Check sheet for the modelled part. Datum: model origin and axes. Units: mm. Coordinates: 2 decimals unless noted, no trailing zeros. Order: outer loops, then holes, each group sorted by start corner. A loop starts at its lowest first (then second) coordinate and runs counter-clockwise, first axis right, second up.
1. Gauge pin test, flat ends, axial feed: pin 1 Ø3 at (x, z) = (46.65, -18) entering from +Y; pin 2 Ø1 at (y, z) = (0.5, 15.5) entering from -X. Record the tip position at first contact, or that the pin passes through.
2. Cross-section at A-A (z = -6). Enter the section's corners in (x, y), then the cut area to 3 significant figures.
3. Thickness scan on line 1 (Z direction, x = 0, y = 1.45); line 2 (X direction, y = 1.35, z = 11.5); line 3 (Z direction, x = 34, y = 0.65). Record the ranges inside material, lowest first.
4. Cross-section at D-D (z = 23). Enter the section's corners in (x, y).
5. Cross-section at C-C (x = 0). Enter the section's corners in (y, z), then the cut area to 3 significant figures.
6. Cross-section at B-B (y = 0.3). Enter the section's corners in (x, z).
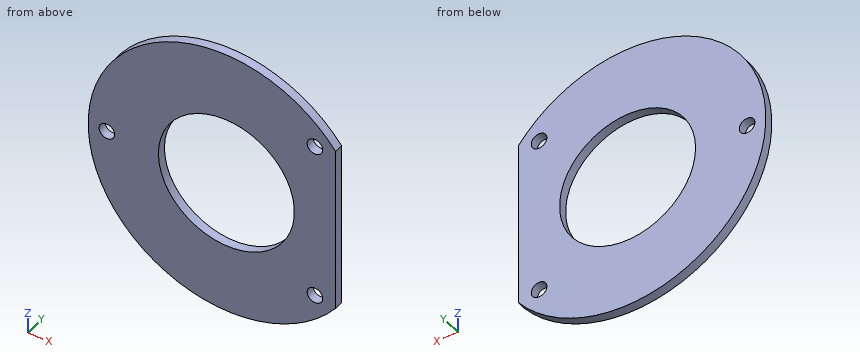
Autodesk Inventor part; units mm, degrees
ref_plane "YZ Plane" through (0, 0, 0) normal (1, 0, 0) x (0, 1, 0)
ref_plane "XZ Plane" through (0, 0, 0) normal (0, 1, 0) x (-1, 0, 0)
ref_plane "XY Plane" through (0, 0, 0) normal (0, 0, 1) x (1, 0, 0)
sketch "Sketch1" plane through (0, 0, 0) normal (0, 1, 0) x (-1, 0, 0)
  circle A0 centre (0, 0) radius 1.75
  line L0 (0, 0) -> (-46.6476, -18) construction
  line L1 (-46.6476, -18) -> (-46.6476, 18) construction
  line L2 (-46.6476, 18) -> (0, 0) construction
  circle A1 centre (-46.6476, -18) radius 1.75 construction
  circle A2 centre (-46.6476, -18) radius 1.75
  circle A3 centre (-46.6476, 18) radius 1.75
  circle A4 centre (-34.2997, 0) radius 12.3479 construction
  arc A5 (0, 0) -> (-46.6476, 18) centre (-26.7967, 0) ccw construction
  arc A6 (-46.6476, 18) -> (-46.6476, -18) centre (-26.7967, 0) ccw construction
  arc A7 (-46.6476, -18) -> (0, 0) centre (-26.7967, 0) ccw construction
  circle A8 centre (-26.7967, 0) radius 31
  circle A9 centre (-26.7967, 0) radius 15.25
  line L3 (-51.2967, 18.9934) -> (-51.2967, -18.9934)
  dimension "d4" = 3.5
  dimension "d5" = 50
  dimension "d6" = 36
  dimension "d7" = 18
  dimension "d8" = 3.5
  dimension "d9" = 3.5
  dimension "d10" = 3.5
  dimension "d11" = 62
  dimension "d12" = 30.5
  dimension "d15" = 24.5
extrude "Extrusion1" add sketch "Sketch1" along normal blind 2 contours A8 L3 picked at (-48.2134, 0)
properties part number "00_Zeiss_Axiotech_Eyepiecemount"
Data:
1. pin 1: passes through
1. pin 2: stops at x = -0.33
2. outline: (-3.62, 0) - (12.78, 0) - (12.78, 2) - (-3.62, 2) - close; (40.82, 0) - (51.3, 0) - (51.3, 2) - (40.82, 2) - close
2. area: 53.7 mm2
3. line 1: z = -15.59 to -1.75, 1.75 to 15.59
3. line 2: x = -1.99 to 16.78, 36.81 to 51.3
3. line 3: z = -30.15 to -13.44, 13.44 to 30.15
4. outline: (6.01, 0) - (47.58, 0) - (47.58, 2) - (6.01, 2) - close
5. outline: (0, -15.59) - (2, -15.59) - (2, -1.75) - (0, -1.75) - close; (0, 1.75) - (2, 1.75) - (2, 15.59) - (0, 15.59) - close
5. area: 55.3 mm2
6. outline: (51.3, -18.99) - (51.3, 18.99) arc R31 ccw (long way) to start; hole circle Ø3.5 at (0, 0); hole circle Ø30.5 at (26.8, 0); hole circle Ø3.5 at (46.65, -18); hole circle Ø3.5 at (46.65, 18)
